Source: CAD feature listing. Evaluate the final solid. Frame: model axes, mm. Face numbers are marked on the shaded views. A direction names the side the tool comes from. Coordinates: 2 decimals unless noted, no trailing zeros. Order: outer loops, then holes, each group sorted by start corner. A loop starts at its lowest first (then second) coordinate and runs counter-clockwise, first axis right, second up. Notation, with made-up numbers: (62, 18.25) -> (112, 18.25) arc R16 cw to (112, 40.25) -> close; hole circle Ø5 at (68.25, 1). An arc over 180 degrees is marked (long way). Write item = value, one per line. Start each with the question number.
Item 1: Section query B-B (y = 9.5). Count the separate pieces of the cut face and the enclosed holes in it, then the cut area to 3 significant figures.
Item 2: Set-up query: the marked faces 1, 2, 3, 4 and 5. Return all of +Z, -Z, +X, -X, +Y, -Y with unobstructed straight access to the full face (end or side cutting, diameter ignored); none if empty.
Item 3: Section query C-C (x = 76.1). Output: boundary loops of the cut face in (y, z), then the cut area to 3 significant figures.
Item 4: Ray query, line 1 along Z through (x, y) = (52, 2.25); line 2 along X through (y, z) = (2.15, -6); line 3 along X through (y, z) = (11.25, -38). Return the intervals inside material, ascending. Write a range as [from, to].
Item 5: Section query A-A (z = -62.5). Output: boundary loops of the cut face in (x, y).
Item 6: Contact query for flat-ended pins moving along their axis: pin 1 (3 mm diameter, centred on x = 28.5, y = 5, fed in from +Z); pin 2 (1.6 mm diameter, centred on x = 63, y = 7.5, fed in from +Z); pin 3 (5.5 mm diameter, centred on x = 8, z = -16.5, fed in from +Y); pin 4 (22 mm diameter, centred on x = 36, z = -78, fed in from +Y). Output: stop coordinate, or through.
Item 7: Mould query, pull axis X, two halves, no side actions, for the marked faces 6, 7 and 8. Classes: released by +X, released by -X, zero draft, split by the parting line, or undercut.
```python
from build123d import *

# Parameters (mm, degrees)
SKETCH1_R           = 1.6
SKETCH1_W           = 25
SKETCH1_H           = 5
SKETCH1_W_2         = 35
SKETCH1_H_2         = 11
BOSS_EXTRUDE1_DEPTH = 4
CHAMFER1_SIZE       = 1.4
SKETCH2_W           = 48
SKETCH2_H           = 9
SKETCH2_R           = 2.075
BOSS_EXTRUDE2_DEPTH = 7
SKETCH3_W           = 11
SKETCH3_H           = 37.5
SKETCH3_R           = 1.6
BOSS_EXTRUDE3_DEPTH = 2
SKETCH4_W           = 5.6
SKETCH4_H           = 8
BOSS_EXTRUDE4_DEPTH = 10.2
SKETCH5_W           = 1.4
SKETCH5_H           = 31.4
BOSS_EXTRUDE5_DEPTH = 2
CUT_EXTRUDE1_DEPTH  = 1
SKETCH8_W           = 26.1
SKETCH8_H           = 5
CUT_EXTRUDE2_DEPTH  = 5.7
SKETCH9_W           = 15.5
SKETCH9_H           = 10
CUT_EXTRUDE3_DEPTH  = 2.25
SKETCH10_W          = 4.6
SKETCH10_H          = 2
SKETCH10_W_2        = 1.9
CUT_EXTRUDE4_DEPTH  = 1.2
SKETCH11_W          = 15.5
SKETCH11_H          = 1
CUT_EXTRUDE5_DEPTH  = 1
SKETCH12_R          = 2.075
CUT_EXTRUDE6_DEPTH  = 7
FILLET1_R           = 2
CUT_EXTRUDE7_REACH  = 97.282
SKETCH14_W          = 16
SKETCH14_H          = 2
BOSS_EXTRUDE6_DEPTH = 1
FILLET2_R           = 0.6


with BuildPart() as part:
    # Sketch1 → Boss-Extrude1 (new body)
    with BuildSketch(Plane(origin=(0, 0, 0), x_dir=(1, 0, 0), z_dir=(0, 1, 0))):
        Polygon((0, 0), (0, 37.5), (17.55, 37.5), (17.55, 86.5), (65.55, 86.5), (65.55, 37.5), (83.1, 37.5), (83.1, 0), align=None)
        with Locations(Location((7, 25.5, 0), (0, 0, 270))):
            Circle(SKETCH1_R, mode=Mode.SUBTRACT)
        with Locations(Location((7, 6, 0), (0, 0, 270))):
            Circle(SKETCH1_R, mode=Mode.SUBTRACT)
        with Locations(Location((76.1, 6, 0), (0, 0, 270))):
            Circle(SKETCH1_R, mode=Mode.SUBTRACT)
        with Locations(Location((76.1, 25.5, 0), (0, 0, 270))):
            Circle(SKETCH1_R, mode=Mode.SUBTRACT)
        with Locations((41.55, 80)):
            Rectangle(SKETCH1_W, SKETCH1_H, mode=Mode.SUBTRACT)
        with Locations((41.55, 64.5)):
            Rectangle(SKETCH1_W_2, SKETCH1_H_2, mode=Mode.SUBTRACT)
    extrude(amount=BOSS_EXTRUDE1_DEPTH)

    # Chamfer1
    chamfer1_edges = [part.edges().sort_by_distance(p)[0] for p in [
        (7, 0, -27.1),
        (7, 0, -7.6),
        (76.1, 0, -7.6),
        (76.1, 0, -27.1),
    ]]
    chamfer(chamfer1_edges, length=CHAMFER1_SIZE)

    # Sketch2 → Boss-Extrude2 (add)
    with BuildSketch(Plane(origin=(0, 4, 0), x_dir=(1, 0, 0), z_dir=(0, 1, 0))):
        with Locations((41.55, 54.5)):
            Rectangle(SKETCH2_W, SKETCH2_H)
        with Locations(Location((23.55, 54.502162277, 0), (0, 0, 270))):
            Circle(SKETCH2_R, mode=Mode.SUBTRACT)
        with Locations(Location((59.55, 54.502162277, 0), (0, 0, 270))):
            Circle(SKETCH2_R, mode=Mode.SUBTRACT)
    extrude(amount=BOSS_EXTRUDE2_DEPTH)

    # Sketch3 → Boss-Extrude3 (add)
    # profile 1 of 2: a face of its own
    with BuildSketch(Plane(origin=(0, 4, 0), x_dir=(1, 0, 0), z_dir=(0, 1, 0))):
        with Locations((5.5, 18.75)):
            Rectangle(SKETCH3_W, SKETCH3_H)
        with Locations(Location((7, 25.5, 0), (0, 0, 90))):
            Circle(SKETCH3_R, mode=Mode.SUBTRACT)
        with Locations(Location((7, 6, 0), (0, 0, 90))):
            Circle(SKETCH3_R, mode=Mode.SUBTRACT)
    # profile 2 of 2: a face of its own
    with BuildSketch(Plane(origin=(0, 4, 0), x_dir=(1, 0, 0), z_dir=(0, 1, 0))):
        with Locations((77.6, 18.75)):
            Rectangle(SKETCH3_W, SKETCH3_H)
        with Locations(Location((76.1, 6, 0), (0, 0, 90))):
            Circle(SKETCH3_R, mode=Mode.SUBTRACT)
        with Locations(Location((76.1, 25.5, 0), (0, 0, 90))):
            Circle(SKETCH3_R, mode=Mode.SUBTRACT)
    extrude(amount=BOSS_EXTRUDE3_DEPTH)

    # Sketch4 → Boss-Extrude4 (add)
    with BuildSketch(Plane(origin=(0, 4, 0), x_dir=(1, 0, 0), z_dir=(0, 1, 0))):
        Polygon((18.27, 42.5), (18.27, 31.4), (21.37, 31.4), (21.37, 40.6), (35.47, 40.6), (35.47, 39.4), (28.97, 39.4), (28.97, 31.4), (34.13, 31.4), (34.13, 29.4), (56.13, 29.4), (56.13, 31.4), (60.73, 31.4), (60.73, 39.4), (54.23, 39.4), (54.23, 40.6), (61.73, 40.6), (61.73, 31.4), (64.83, 31.4), (64.83, 44.4), (25.1, 44.4), (25.1, 42.5), align=None)
        with Locations((25.17, 35.4)):
            Rectangle(SKETCH4_W, SKETCH4_H)
    extrude(amount=BOSS_EXTRUDE4_DEPTH)

    # Sketch5 → Boss-Extrude5 (add)
    with BuildSketch(Plane(origin=(0, 4, 0), x_dir=(1, 0, 0), z_dir=(0, 1, 0))):
        with Locations((20.67, 15.7)):
            Rectangle(SKETCH5_W, SKETCH5_H)
        with Locations((23.07, 15.7)):
            Rectangle(SKETCH5_W, SKETCH5_H)
        with Locations((60.03, 15.7)):
            Rectangle(SKETCH5_W, SKETCH5_H)
        with Locations((62.43, 15.7)):
            Rectangle(SKETCH5_W, SKETCH5_H)
    extrude(amount=BOSS_EXTRUDE5_DEPTH)

    # Sketch7 → Cut-Extrude1 (cut)
    with BuildSketch(Plane(origin=(0, 4, 0), x_dir=(1, 0, 0), z_dir=(0, 1, 0))):
        Polygon((28.97, 31.4), (28.97, 18.4), (27.97, 18.4), (27.97, 31.4), (27.97, 39.4), (22.37, 39.4), (22.37, 0), (21.37, 0), (21.37, 40.6), (35.47, 40.6), (35.47, 39.4), (28.97, 39.4), align=None)
        Polygon((60.73, 0), (61.73, 0), (61.73, 40.6), (54.23, 40.6), (54.23, 39.4), (60.73, 39.4), align=None)
    extrude(amount=-CUT_EXTRUDE1_DEPTH, mode=Mode.SUBTRACT)

    # Sketch8 → Cut-Extrude2 (cut)
    with BuildSketch(Plane(origin=(0, 14.2, 0), x_dir=(1, 0, 0), z_dir=(0, 1, 0))):
        Polygon((35.47, 40.6), (35.47, 44.4), (25.1, 44.4), (25.1, 42.5), (21.37, 42.5), (21.37, 40.6), align=None)
        with Locations((51.78, 41.9)):
            Rectangle(SKETCH8_W, SKETCH8_H)
    extrude(amount=-CUT_EXTRUDE2_DEPTH, mode=Mode.SUBTRACT)

    # Sketch9 → Cut-Extrude3 (cut)
    with BuildSketch(Plane(origin=(0, 14.2, 0), x_dir=(1, 0, 0), z_dir=(0, 1, 0))):
        with Locations((46.48, 34.4)):
            Rectangle(SKETCH9_W, SKETCH9_H)
    extrude(amount=-CUT_EXTRUDE3_DEPTH, mode=Mode.SUBTRACT)

    # Sketch10 → Cut-Extrude4 (cut)
    with BuildSketch(Plane(origin=(0, 14.2, 0), x_dir=(1, 0, 0), z_dir=(0, 1, 0))):
        with Locations((36.43, 30.4)):
            Rectangle(SKETCH10_W, SKETCH10_H)
        with Locations((55.18, 30.4)):
            Rectangle(SKETCH10_W_2, SKETCH10_H)
    extrude(amount=-CUT_EXTRUDE4_DEPTH, mode=Mode.SUBTRACT)

    # Sketch11 → Cut-Extrude5 (cut)
    with BuildSketch(Plane(origin=(0, 11.95, 0), x_dir=(1, 0, 0), z_dir=(0, 1, 0))):
        with Locations((46.48, 29.9)):
            Rectangle(SKETCH11_W, SKETCH11_H)
    extrude(amount=-CUT_EXTRUDE5_DEPTH, mode=Mode.SUBTRACT)

    # Sketch12 → Cut-Extrude6 (cut)
    with BuildSketch(Plane(origin=(0, 11.95, 0), x_dir=(1, 0, 0), z_dir=(0, 1, 0))):
        with Locations(Location((46.5, 35.4, 0), (0, 0, 270))):
            Circle(SKETCH12_R)
    extrude(amount=-CUT_EXTRUDE6_DEPTH, mode=Mode.SUBTRACT)

    # Fillet1
    fillet1_edges = [part.edges().sort_by_distance(p)[0] for p in [
        (38.73, 11.35, -44.4),
    ]]
    fillet(fillet1_edges, radius=FILLET1_R)

    # Sketch13 → Cut-Extrude7 (cut, up to next)
    with BuildSketch(Plane(origin=(0, 0, -44.4), x_dir=(-1, 0, 0), z_dir=(0, 0, -1)), mode=Mode.PRIVATE) as cut_extrude7_sk1:
        with BuildLine():
            Line((-58.73, 8.5), (-58.73, 5.57))
            ThreePointArc((-58.73, 5.57), (-57.38, 4.22), (-56.03, 5.57))
            Line((-56.03, 5.57), (-56.03, 8.5))
            Line((-56.03, 8.5), (-58.73, 8.5))
        make_face()
    cut_extrude7_tool1 = extrude(cut_extrude7_sk1.sketch, amount=-CUT_EXTRUDE7_REACH, mode=Mode.PRIVATE) & part.part
    # Sketch13 → Cut-Extrude7 (cut, up to next)
    with BuildSketch(Plane(origin=(0, 0, -44.4), x_dir=(-1, 0, 0), z_dir=(0, 0, -1)), mode=Mode.PRIVATE) as cut_extrude7_sk2:
        with BuildLine():
            Line((-33.57, 8.5), (-33.57, 6.8))
            ThreePointArc((-33.57, 6.8), (-32.22, 5.45), (-30.87, 6.8))
            Line((-30.87, 6.8), (-30.87, 8.5))
            Line((-30.87, 8.5), (-33.57, 8.5))
        make_face()
    cut_extrude7_tool2 = extrude(cut_extrude7_sk2.sketch, amount=-CUT_EXTRUDE7_REACH, mode=Mode.PRIVATE) & part.part
    # Sketch13 → Cut-Extrude7 (cut, up to next)
    with BuildSketch(Plane(origin=(0, 0, -44.4), x_dir=(-1, 0, 0), z_dir=(0, 0, -1)), mode=Mode.PRIVATE) as cut_extrude7_sk3:
        with BuildLine():
            Line((-26.49, 5.57), (-26.49, 8.5))
            Line((-26.49, 8.5), (-23.79, 8.5))
            Line((-23.79, 8.5), (-23.79, 5.57))
            ThreePointArc((-23.79, 5.57), (-25.14, 4.22), (-26.49, 5.57))
        make_face()
    cut_extrude7_tool3 = extrude(cut_extrude7_sk3.sketch, amount=-CUT_EXTRUDE7_REACH, mode=Mode.PRIVATE) & part.part
    add(cut_extrude7_tool1.solids().sort_by_distance((57.38, 6.49348, -44.4))[0], mode=Mode.SUBTRACT)
    add(cut_extrude7_tool2.solids().sort_by_distance((32.22, 7.10341, -44.4))[0], mode=Mode.SUBTRACT)
    add(cut_extrude7_tool3.solids().sort_by_distance((25.14, 6.49348, -44.4))[0], mode=Mode.SUBTRACT)

    # Sketch14 → Boss-Extrude6 (add)
    with BuildSketch(Plane(origin=(0, 4, 0), x_dir=(1, 0, 0), z_dir=(0, 1, 0))):
        with Locations((41.55, 1)):
            Rectangle(SKETCH14_W, SKETCH14_H)
    extrude(amount=BOSS_EXTRUDE6_DEPTH)

    # Fillet2
    fillet2_edges = [part.edges().sort_by_distance(p)[0] for p in [
        (41.55, 5, 0),
        (41.55, 5, -2),
    ]]
    fillet(fillet2_edges, radius=FILLET2_R)


solid = part.part
```
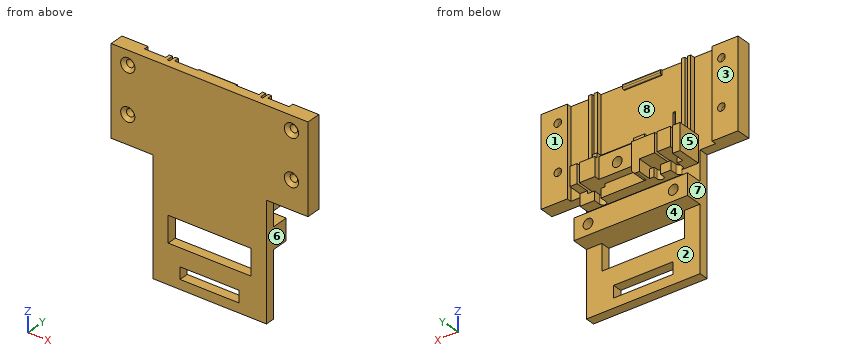
Computed:
q1.separate_pieces = 5
q1.enclosed_holes = 3
q1.area = 809 mm^2
q2.face_1 = +Z, -Z, +X, +Y
q2.face_2 = -Z, +X, -X, +Y
q2.face_3 = +Z, -Z, -X, +Y
q2.face_4 = +Y
q2.face_5 = +Z, +Y
q3.outline = (0, -37.5) -> (6, -37.5) -> (6, -27.1) -> (1.4, -27.1) -> (0, -28.5) -> close; (0, -22.5) -> (1.4, -23.9) -> (6, -23.9) -> (6, -7.6) -> (1.4, -7.6) -> (0, -9) -> close; (0, -3) -> (1.4, -4.4) -> (6, -4.4) -> (6, 0) -> (0, 0) -> close
q3.area = 183 mm^2
q4.line_1 = [-86.5, -82.5], [-77.5, -70], [-59, 0]
q4.line_2 = [0, 5.4], [8.6, 74.5], [77.7, 83.1]
q4.line_3 = [18.27, 21.37], [22.37, 27.97], [28.97, 60.73], [61.73, 64.83]
q5.outline = (17.55, 0) -> (24.05, 0) -> (24.05, 4) -> (17.55, 4) -> close; (59.05, 0) -> (65.55, 0) -> (65.55, 4) -> (59.05, 4) -> close
q6.pin_1 = 0
q6.pin_2 = -31.4
q6.pin_3 = 6
q6.pin_4 = 4
q7.face_6 = released by +X
q7.face_7 = released by -X
q7.face_8 = undercut
